from build123d import *

# Parameters (mm, degrees)
SKETCH1_R           = 12.5
BOSS_EXTRUDE1_DEPTH = 40
SKETCH2_W           = 25
SKETCH2_H           = 35
BOSS_EXTRUDE2_DEPTH = 30
SKETCH3_W           = 25
SKETCH3_H           = 20
CUT_EXTRUDE1_DEPTH  = 77.362621747
FILLET1_R           = 5
SKETCH4_R           = 7.5
CUT_EXTRUDE2_DEPTH  = 65


with BuildPart() as part:
    # Sketch1 → Boss-Extrude1 (new body)
    with BuildSketch(Plane(origin=(0, 0, 0), x_dir=(1, 0, 0), z_dir=(0, 1, 0))):
        with Locations(Location((0, 0, 0), (0, 0, 270))):
            Circle(SKETCH1_R)
    extrude(amount=BOSS_EXTRUDE1_DEPTH)

    # Sketch2 → Boss-Extrude2 (add)
    with BuildSketch(Plane(origin=(0, 40, 0), x_dir=(1, 0, 0), z_dir=(0, 1, 0))):
        Rectangle(SKETCH2_W, SKETCH2_H)
    extrude(amount=BOSS_EXTRUDE2_DEPTH)

    # Sketch3 → Cut-Extrude1 (cut, through all)
    with BuildSketch(Plane(origin=(12.5, 0, 0), x_dir=(0, 0, -1), z_dir=(1, 0, 0))):
        with Locations((0, 55)):
            Rectangle(SKETCH3_W, SKETCH3_H)
    extrude(amount=-CUT_EXTRUDE1_DEPTH, mode=Mode.SUBTRACT)

    # Fillet1
    fillet1_edges = [part.edges().sort_by_distance(p)[0] for p in [
        (0, 40, 17.5),
        (0, 40, -17.5),
        (0, 70, 17.5),
        (0, 70, -17.5),
    ]]
    fillet(fillet1_edges, radius=FILLET1_R - 0.0001)  # a hair under: the kernel refuses the full size

    # Sketch4 → Cut-Extrude2 (cut)
    with BuildSketch(Plane.XZ):
        with Locations(Location((0, 0, 0), (0, 0, 270))):
            Circle(SKETCH4_R)
    extrude(amount=-CUT_EXTRUDE2_DEPTH, mode=Mode.SUBTRACT)


solid = part.part
Could you check a few things on this model? Use its own coordinates, in mm. A direction names the side the tool comes from. Coordinates: 2 decimals unless noted, no trailing zeros. Order: outer loops, then holes, each group sorted by start corner. A loop starts at its lowest first (then second) coordinate and runs counter-clockwise, first axis right, second up.
Q1. Please list where these lines run through material, in increasing order: L1, parallel to Z at x = -1, y = 53.5; L2, parallel to Y at x = 3.5, z = -9; L3, parallel to Y at x = -7.5, z = -12.
Q2. Will these pins go through, and if not, where does the flat tip stop? pin 1 (1.5 mm diameter, centred on y = 33.5, z = 8, fed in from +X); pin 2 (8 mm diameter, centred on x = 2, y = 7.5, fed in from -Z); pin 3 (3 mm diameter, centred on x = 3.5, y = 19, fed in from +Z).
Q3. Suppose I cut it at C-C on z = 5. Please give me the cut outline in (x, y), and give its area (3 significant figures).
Q4. Suppose I cut it at B-B on y = 61. Please give me the cut outline in (x, z).
Q5. Suppose I cut it at A-A on z = -10. Please give me the cut outline in (x, y).
Q6. Thinking about a two-plate mould opening in Z: for faces 1 (the cylindrical face through (0.18, 68.57, -16)), 2 (the flat face through (-12.5, 44.8, 0.2)), 3 (the flat face through (6, 45, 6)), which applies, released by +Z, released by -Z, zero draft, split by the parting line, or undercut?
Q7. Which directions (+Z, -Z, +X, -X, +Y, -Y) give clear straight access to the entire face, cutting with the end or side of a thin tool? Please do faces 4 (the flat face through (-3.8, 40, -12.3)), 5 (the flat face through (0, 65, 0)), 6 (the cylindrical face through (3.755, 19.72, 11.923)).
Answer:
1. L1: z = -17.5 to -12.5, 12.5 to 17.5
1. L2: y = 0 to 45, 65 to 70
1. L3: y = 40 to 45, 65 to 70
2. pin 1: stops at x = 10.18
2. pin 2: stops at z = -12.5
2. pin 3: stops at z = 12.34
3. outline: (-12.5, 40) - (-11.46, 40) - (-11.46, 0) - (-5.59, 0) - (-5.59, 45) - (-12.5, 45) - close; (-12.5, 65) - (12.5, 65) - (12.5, 70) - (-12.5, 70) - close; (5.59, 0) - (11.46, 0) - (11.46, 40) - (12.5, 40) - (12.5, 45) - (5.59, 45) - close
3. area: 663 mm2
4. outline: (-12.5, -17.5) - (12.5, -17.5) - (12.5, -12.5) - (-12.5, -12.5) - close; (-12.5, 12.5) - (12.5, 12.5) - (12.5, 17.5) - (-12.5, 17.5) - close
5. outline: (-12.5, 40) - (-7.5, 40) - (-7.5, 0) - (7.5, 0) - (7.5, 40) - (12.5, 40) - (12.5, 45) - (-12.5, 45) - close; (-12.5, 65) - (12.5, 65) - (12.5, 70) - (-12.5, 70) - close
6. face 1: released by -Z
6. face 2: zero draft
6. face 3: undercut
7. face 4: -Z, -Y
7. face 5: +X, -X
7. face 6: -Y
